Can you work these out from the model? Positions are in its coordinate system, mm. Face numbers are marked on the shaded views. A direction names the side the tool comes from. Round coordinates to 2 decimals unless told otherwise and drop trailing zeros. Order: outer loops, then holes, each group sorted by start corner. A loop starts at its lowest first (then second) coordinate and runs counter-clockwise, first axis right, second up. Notation, with made-up numbers: M 8.25,-14.75 L 37.25,-14.75 A19 cw 37.25,17.25 Z; hole C 62,63 d10. An arc over 180 degrees is marked long. Answer as CSV lines item,"result". Start each with the question number.
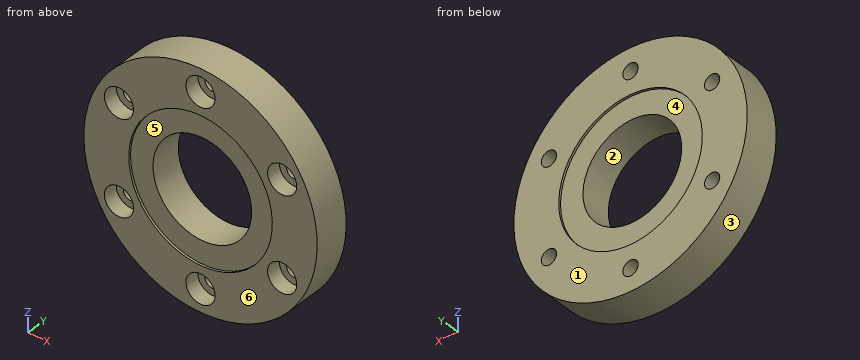
from build123d import *

# Parameters (mm, degrees)
SKETCH_1_R          = 26
SKETCH_1_R_2        = 1.7
SKETCH_1_R_3        = 16
EXTRUDE_1_DEPTH     = 8
SKETCH_2_R          = 3.25
CUT_EXTRUDE_1_DEPTH = 3.3
EXTRUDE_START       = 0.5
SKETCH_3_R          = 16
SKETCH_3_R_2        = 11
EXTRUDE_2_DEPTH     = 7


with BuildPart() as part:
    # 草图1 → 凸台-拉伸1 (new body)
    with BuildSketch(Plane(origin=(0, 0, 0), x_dir=(1, 0, 0), z_dir=(0, 1, 0))):
        with Locations(Location((0, 0, 0), (0, 0, 270))):
            Circle(SKETCH_1_R)
        with Locations(Location((0, 21, 0), (0, 0, 270))):
            Circle(SKETCH_1_R_2, mode=Mode.SUBTRACT)
        with Locations(Location((18.186533479, 10.5, 0), (0, 0, 270))):
            Circle(SKETCH_1_R_2, mode=Mode.SUBTRACT)
        with Locations(Location((18.186533479, -10.5, 0), (0, 0, 270))):
            Circle(SKETCH_1_R_2, mode=Mode.SUBTRACT)
        with Locations(Location((0, -21, 0), (0, 0, 270))):
            Circle(SKETCH_1_R_2, mode=Mode.SUBTRACT)
        with Locations(Location((-18.186533479, -10.5, 0), (0, 0, 270))):
            Circle(SKETCH_1_R_2, mode=Mode.SUBTRACT)
        with Locations(Location((-18.186533479, 10.5, 0), (0, 0, 270))):
            Circle(SKETCH_1_R_2, mode=Mode.SUBTRACT)
        with Locations(Location((0, 0, 0), (0, 0, 270))):
            Circle(SKETCH_1_R_3, mode=Mode.SUBTRACT)
    extrude(amount=EXTRUDE_1_DEPTH)

    # 草图2 → 切除-拉伸1 (cut)
    with BuildSketch(Plane(origin=(0, 0, 0), x_dir=(1, 0, 0), z_dir=(0, 1, 0))):
        with Locations(Location((0, 21, 0), (0, 0, 270))):
            Circle(SKETCH_2_R)
        with Locations(Location((18.186533479, 10.5, 0), (0, 0, 270))):
            Circle(SKETCH_2_R)
        with Locations(Location((18.186533479, -10.5, 0), (0, 0, 270))):
            Circle(SKETCH_2_R)
        with Locations(Location((0, -21, 0), (0, 0, 270))):
            Circle(SKETCH_2_R)
        with Locations(Location((-18.186533479, -10.5, 0), (0, 0, 270))):
            Circle(SKETCH_2_R)
        with Locations(Location((-18.186533479, 10.5, 0), (0, 0, 270))):
            Circle(SKETCH_2_R)
    extrude(amount=CUT_EXTRUDE_1_DEPTH, mode=Mode.SUBTRACT)

    # 草图3 → 凸台-拉伸2 (add)
    with BuildSketch(Plane(origin=(0, 0, 0), x_dir=(1, 0, 0), z_dir=(0, 1, 0)).offset(EXTRUDE_START)):
        with Locations(Location((0, 0, 0), (0, 0, 270))):
            Circle(SKETCH_3_R)
        with Locations(Location((0, 0, 0), (0, 0, 270))):
            Circle(SKETCH_3_R_2, mode=Mode.SUBTRACT)
    extrude(amount=EXTRUDE_2_DEPTH)


solid = part.part
(1) I want a section at D-D on x = -13. Write out the boundary of the cut face in (y, z).
(2) I want a section at C-C on z = 10. Count the separate pieces of the cut face and the enclosed holes in it, and give its area (3 significant figures).
(3) If we mould it in two halves opening along Z, with no side actions, what happens to the marked faces 1, 2 and 3? For each: +Z half, -Z half, draft (parallel to the pull), parting line (faces both ways), or undercut.
(4) If I drill on line 1 along Z through (x, y) = (-16, 2.5); line 2 along Z through (x, y) = (3, 2.5); line 3 along Z through (x, y) = (-1, 5), over which ranges is the centre line in solid material (lowest first)?
(5) I'm going to push flat-ended pins straight in: P1, Ø5.5, axis at x = -18.19, z = 10.5, coming from the -Y side; P2, Ø4, axis at x = 18.19, z = -10.5, coming from the +Y side; P3, Ø9.5, axis at x = 6.5, z = 0.5, coming from the -Y side; P4, Ø2, axis at x = -1.5, y = 5.5, coming from the -Z side. Where does each tip first touch, or does it pass through?
(6) I want a section at B-B on y = 1.25. Write out the boundary of the cut face in (x, z), and give its area (3 significant figures).
(7) I want a section at A-A on z = 0. Write out the boundary of the cut face in (x, y).
(8) For the marked faces 4, 5 and 6, which set-ups out of +Z, -Z, +X, -X, +Y, -Y let a thin tool reach every point of the face, with its end or its side?
From the geometry:
1,outline,"M 0,-22.52 L 8,-22.52 L 8,-9.33 L 7.5,-9.33 L 7.5,9.33 L 8,9.33 L 8,22.52 L 0,22.52 L 0,9.33 L 0.5,9.33 L 0.5,-9.33 L 0,-9.33 Z"
2,separate pieces,"4"
2,enclosed holes,"0"
2,area,"222 mm²"
3,face 1,"draft"
3,face 2,"undercut"
3,face 3,"parting line"
4,line 1,"-20.49 to -12.9, -8.1 to 8.1, 12.9 to 20.49"
4,line 2,"-25.83 to -22.25, -19.75 to -10.58, 10.58 to 19.75, 22.25 to 25.83"
4,line 3,"-25.98 to -22.37, -19.63 to -10.95, 10.95 to 19.63, 22.37 to 25.98"
5,P1,"y = 3.3"
5,P2,"y = 8"
5,P3,"y = 0.5"
5,P4,"z = -26"
6,outline,"C 0,0 d52; hole C -18.19,-10.5 d6.5; hole C -18.19,10.5 d6.5; hole C 0,0 d22; hole C 0,-21 d6.5; hole C 0,21 d6.5; hole C 18.19,-10.5 d6.5; hole C 18.19,10.5 d6.5"
6,area,"1,540 mm²"
7,outline,"M -26,0 L -16,0 L -16,0.5 L -11,0.5 L -11,7.5 L -16,7.5 L -16,8 L -26,8 Z; M 11,0.5 L 16,0.5 L 16,0 L 26,0 L 26,8 L 16,8 L 16,7.5 L 11,7.5 Z"
8,face 4,"+Y"
8,face 5,"-Y"
8,face 6,"+Z, -Z, +X, -X, -Y"
